```python
from build123d import *

# Parameters (mm, degrees)
F0_R     = 2
F1_DEPTH = 5
F3_DEPTH = 5
F5_DEPTH = 5
F6_SIZE  = 2


# Not quite as in the source:
# - a feature names something its author has since deleted; it is built from what else it names


with BuildPart() as f1:
    # F0 (on Top) → F1 (new body)
    with BuildSketch(Plane.XY):
        Polygon((-67.5038768748, 35.6870033689), (-97.5038768748, 35.6870033689), (-97.5038768748, 30.6870033689), (-97.5038768748, 0.6870033689), (-97.5038768748, -4.3129966311), (-67.5038768748, -4.3129966311), align=None)
        with Locations((-90.0038768748, 15.6870033689)):
            Circle(F0_R, mode=Mode.SUBTRACT)
        with Locations((-75.0038768748, 15.6870033689)):
            Circle(F0_R, mode=Mode.SUBTRACT)
    extrude(amount=F1_DEPTH)

    # F2 (on face) → F3 (join)
    with BuildSketch(Plane.XZ.offset(4.3129966311)):
        Polygon((-97.5038768748, 5), (-67.5038768748, 5), (-92.5038768748, 40), (-97.5038768748, 40), align=None)
    extrude(amount=-F3_DEPTH)

    # F4 (on face) → F5 (join)
    with BuildSketch(Plane(origin=(0, 35.6870033689, 0), x_dir=(-1, 0, 0), z_dir=(0, 1, 0))):
        Polygon((92.5038768748, 40), (67.5038768748, 5), (97.5038768748, 5), (97.5038768748, 40), align=None)
    extrude(amount=-F5_DEPTH)

    # F6
    f6_edges = [f1.edges().sort_by_distance(p)[0] for p in [
        (-77.003877, 15.687003, 5),
        (-92.003877, 15.687003, 5),
    ]]
    chamfer(f6_edges, length=F6_SIZE)


solid = f1.part
```
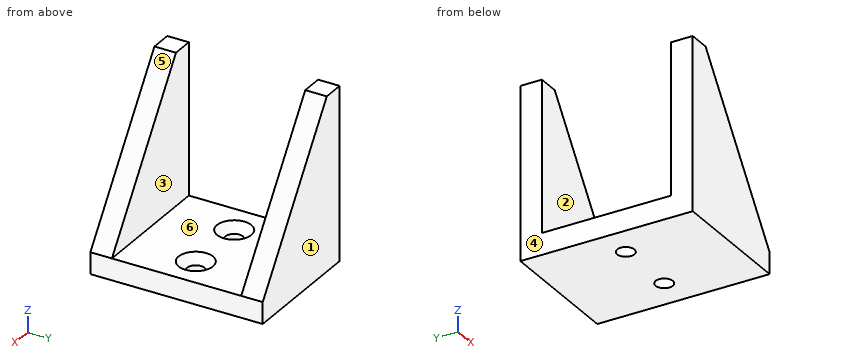
Work out the finished part from the listing and answer in its coordinate system (mm). Face numbers are marked on the shaded views. A direction names the side the tool comes from. Coordinates: 2 decimals unless noted, no trailing zeros. Loops run counter-clockwise (first coordinate to the right, second up) from the corner with the lowest first, then second, coordinate; pieces in that order, holes last. Notation, with made-up numbers: M 75.25,7.5 L 93.25,7.5 A20 cw 93.25,31.5 Z; hole C 71.5,-5 d6. An arc over 180 degrees is marked long. Use CSV: the item, a comma, the result in double quotes. Start each with the question number.
(1) Consider line 1 (Y direction, x = -87, z = 19); line 2 (Z direction, x = -83, y = 15.5); line 3 (X direction, y = 33, z = 29.5). Determine where each line is inside the solid, lowest interval first.
(2) Find section B-B, the plane y = 0. Give the vertices of the cut face in (x, z).
(3) Given pin 1 Ø2 at (x, y) = (-83, 14) entering from +Z; pin 2 Ø12 at (x, y) = (-89.5, 4.5) entering from +Z, each flat-ended and moving along its own axis, determine where each tip first touches the part or whether it passes through.
(4) Find section A-A, the plane z = 34.5. Give the vertices of the cut face in (x, y), then the cut area to 3 significant figures.
(5) For a pull along Y with two mould halves and no side action, classify the marked faces 1, 2, 3 and 4 as +Y half, -Y half, draft (parallel to the pull), parting line (faces both ways), or undercut.
(6) Find section D-D, the plane z = 8.5. Give the vertices of the cut face in (x, y).
(7) Find section C-C, the plane x = -81.75. Give the vertices of the cut face in (y, z), then the cut area to 3 significant figures.
(8) For the marked faces 5 and 6, determine the directions among +Z, -Z, +X, -X, +Y, -Y from which every point of the face is accessible in a straight line to the end or side of a thin tool.
Recorded:
1,line 1,"y = -4.31 to 0.69, 30.69 to 35.69"
1,line 2,"z = 0 to 5"
1,line 3,"x = -97.5 to -85"
2,outline,"M -97.5,0 L -67.5,0 L -67.5,5 L -92.5,40 L -97.5,40 Z"
3,pin 1,"stops at z = 5"
3,pin 2,"stops at z = 40"
4,outline,"M -97.5,-4.31 L -88.58,-4.31 L -88.58,0.69 L -97.5,0.69 Z; M -97.5,30.69 L -88.58,30.69 L -88.58,35.69 L -97.5,35.69 Z"
4,area,"89.3 mm^2"
5,face 1,"+Y half"
5,face 2,"undercut"
5,face 3,"undercut"
5,face 4,"draft"
6,outline,"M -97.5,-4.31 L -70,-4.31 L -70,0.69 L -97.5,0.69 Z; M -97.5,30.69 L -70,30.69 L -70,35.69 L -97.5,35.69 Z"
7,outline,"M -4.31,0 L 35.69,0 L 35.69,24.94 L 30.69,24.94 L 30.69,5 L 0.69,5 L 0.69,24.94 L -4.31,24.94 Z"
7,area,"399 mm^2"
8,face 5,"+Z, +X, +Y, -Y"
8,face 6,"+Z, +X, -X"
